Verification items for the finished model (mm, model axes). Face numbers are marked on the shaded views. Give positions to 0.01 mm unless a question says otherwise; leave off trailing zeros. Loops run counter-clockwise (first coordinate to the right, second up) from the corner with the lowest first, then second, coordinate; pieces in that order, holes last. Notation, with made-up numbers: (25.25, 69) - (69.25, 69) arc R27 ccw to (69.25, 101) - close; hole circle Ø5 at (22.25, 77). An arc over 180 degrees is marked (long way). Use one line per item in the form item = value.
Autodesk Inventor part; units mm, degrees
ref_plane "YZ Plane" through (0, 0, 0) normal (1, 0, 0) x (0, 1, 0)
ref_plane "XZ Plane" through (0, 0, 0) normal (0, 1, 0) x (-1, 0, 0)
ref_plane "XY Plane" through (0, 0, 0) normal (0, 0, 1) x (1, 0, 0)
sketch "Sketch1" plane through (0, 0, 0) normal (0, 1, 0) x (-1, 0, 0)
  circle A0 centre (0, 0) radius 25.9
  circle A1 centre (0, 0) radius 25
  circle A2 centre (0, 0) radius 26.8
  dimension "d0" = 51.8
  dimension "d1" = 50
  dimension "d2" = 53.6
extrude "Extrusion1" add sketch "Sketch1" along normal blind 95 and the other way blind 85 contours A0
extrude "Extrusion2" add sketch "Sketch1" along normal mid plane 180 contours A2
properties part number "payloadchamber" material "ABS Plastic"
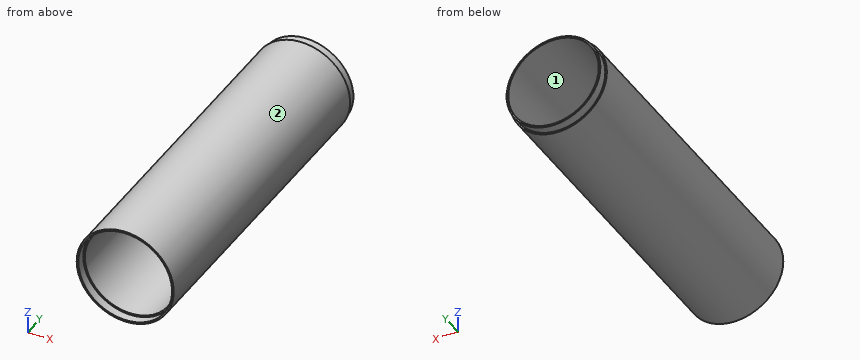
1. Scan lines: probe 1 along Z at (x, y) = (0, -22); probe 2 along Z at (x, y) = (-22.5, 66); probe 3 along X at (y, z) = (19, 1.5). Record each from-to range of solid material in increasing order.
Result set:
probe_1 = -26.8 to -25, 25 to 26.8
probe_2 = -14.56 to -10.9, 10.9 to 14.56
probe_3 = -26.76 to -24.95, 24.95 to 26.76
2. Draft check along X on the marked faces 1 and 2. Enter one of: released by +X, released by -X, zero draft, split by the parting line, or undercut.
Result set:
face_1 = undercut
face_2 = split by the parting line
3. Section check B-B, the plane z = 0. Record the cut outline in (x, y), then the cut area to 3 significant figures.
Result set:
outline = (-26.8, -90) - (-25.9, -90) - (-25.9, -85) - (-25, -85) - (-25, 95) - (-25.9, 95) - (-25.9, 90) - (-26.8, 90) - close; (25, -85) - (25.9, -85) - (25.9, -90) - (26.8, -90) - (26.8, 90) - (25.9, 90) - (25.9, 95) - (25, 95) - close
area = 648 mm²
4. Section check C-C, the plane y = -39. Record the cut outline in (x, z), then the cut area to 3 significant figures.
Result set:
outline = circle Ø53.6 at (0, 0); hole circle Ø50 at (0, 0)
area = 293 mm²
5. Section check A-A, the plane x = 0. Record the cut outline in (y, z), then the cut area to 3 significant figures.
Result set:
outline = (-90, -26.8) - (90, -26.8) - (90, -25.9) - (95, -25.9) - (95, -25) - (-85, -25) - (-85, -25.9) - (-90, -25.9) - close; (-90, 25.9) - (-85, 25.9) - (-85, 25) - (95, 25) - (95, 25.9) - (90, 25.9) - (90, 26.8) - (-90, 26.8) - close
area = 648 mm²
6. Depth check by flat-ended pin: pin 1 Ø2 at (x, y) = (-5.5, 3.5) entering from +Z; pin 2 Ø1.5 at (y, z) = (24, -10.5) entering from +X; pin 3 Ø3 at (x, y) = (-18.5, 39) entering from +Z. Enter the tip coordinate at first touch or a pass-through.
Result set:
pin_1 = 26.42
pin_2 = 24.96
pin_3 = 20.72
